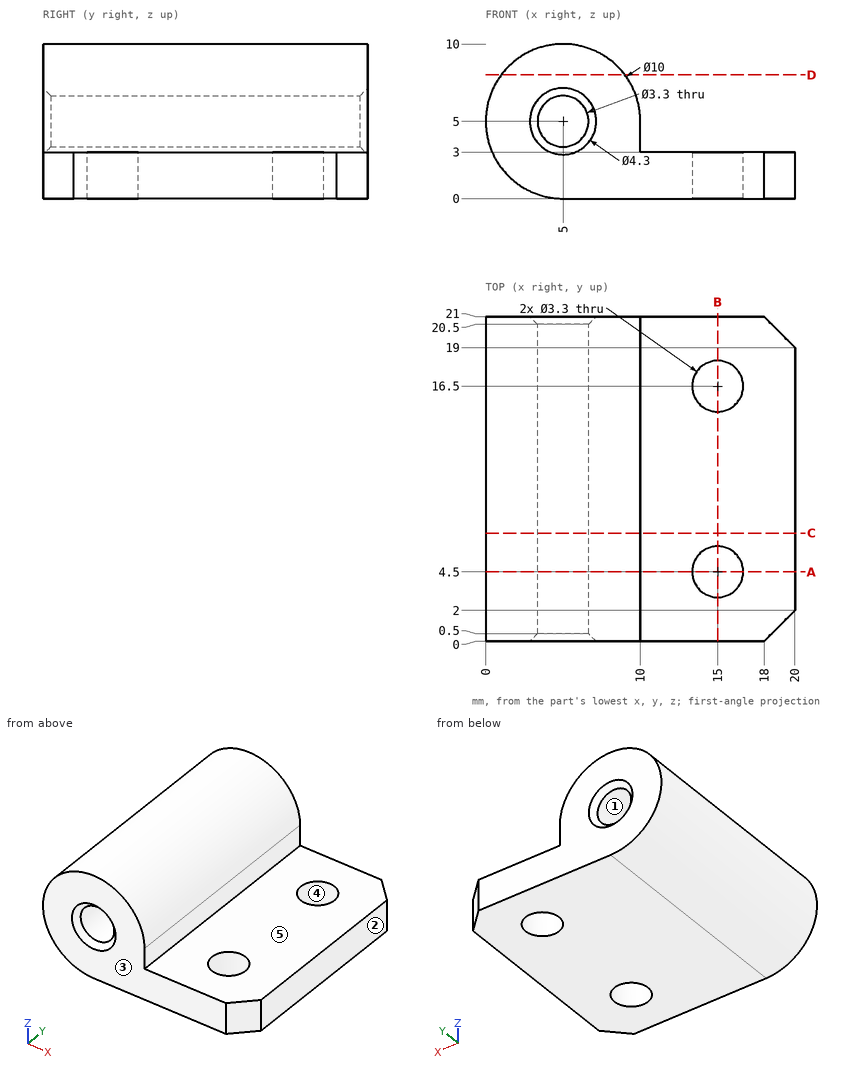
Check sheet for the drawn part. Datum: minimum x, y, z corner. Units: mm. A direction names the side the tool comes from. Give positions to 0.01 mm unless a question says otherwise; leave off trailing zeros. Loops run counter-clockwise (first coordinate to the right, second up) from the corner with the lowest first, then second, coordinate; pieces in that order, holes last.
1) Sectioned sample at A-A, the plane y = 4.5. Enter the section's corners in (x, z), then the cut area to 3 significant figures.
2) Depth check by flat-ended pin: pin 1 Ø4 at (x, y) = (15, 4.5) entering from +Z; pin 2 Ø2 at (x, y) = (15, 16.5) entering from +Z; pin 3 Ø4 at (x, z) = (10.5, 4) entering from -Y; pin 4 Ø0.6 at (y, z) = (9, 4.5) entering from +X. Enter the tip coordinate at first touch or a pass-through.
3) Sectioned sample at B-B, the plane x = 15. Enter the section's corners in (y, z).
4) Draft check along X on the marked faces 1, 2 and 3. Enter one of: pulls with the +X half, pulls with the -X half, needs draft (parallel to the pull), parting line crosses it, or undercut.
5) Thickness scan on line 1 along Y through (x, z) = (15, 1.75); line 2 along Y through (x, z) = (13.5, 2.75); line 3 along Z through (x, y) = (5.25, 18.25). Record the ranges inside material, lowest first.
6) Set-up check for the marked faces 4 and 5: record each of +Z, -Z, +X, -X, +Y, -Y from which the full face is reachable in a straight line by a thin tool's end or side.
7) Sectioned sample at D-D, the plane z = 8. Enter the section's corners in (x, y), then the cut area to 3 significant figures.
8) Sectioned sample at C-C, the plane y = 7. Enter the section's corners in (x, z).
Answers:
1. outline: (5, 0) - (13.35, 0) - (13.35, 3) - (10, 3) - (10, 5) arc R5 ccw (long way) to start; (16.65, 0) - (20, 0) - (20, 3) - (16.65, 3) - close; hole circle Ø3.3 at (5, 5)
1. area: 95.5 mm2
2. pin 1: stops at z = 3
2. pin 2: passes through
2. pin 3: stops at y = 0
2. pin 4: stops at x = 10
3. outline: (0, 0) - (2.85, 0) - (2.85, 3) - (0, 3) - close; (6.15, 0) - (14.85, 0) - (14.85, 3) - (6.15, 3) - close; (18.15, 0) - (21, 0) - (21, 3) - (18.15, 3) - close
4. face 1: undercut
4. face 2: pulls with the +X half
4. face 3: needs draft
5. line 1: y = 0 to 2.85, 6.15 to 14.85, 18.15 to 21
5. line 2: y = 0 to 3.81, 5.19 to 15.81, 17.19 to 21
5. line 3: z = 0 to 3.37, 6.63 to 9.99
6. face 4: +Z, -Z
6. face 5: +Z, +X, +Y, -Y
7. outline: (1, 0) - (9, 0) - (9, 21) - (1, 21) - close
7. area: 168 mm2
8. outline: (5, 0) - (20, 0) - (20, 3) - (10, 3) - (10, 5) arc R5 ccw (long way) to start; hole circle Ø3.3 at (5, 5)
